Geometry check sheet. Reference: the model listing, model coordinates, mm. Face numbers are marked on the shaded views. A direction names the side the tool comes from. Coordinates: 2 decimals unless noted, no trailing zeros. Write each loop counter-clockwise with the first axis right and the second up, starting at its lowest first coordinate (ties: lowest second). Pieces come first, ordered by that corner, then holes. Notation, with made-up numbers: (30, 66.5) -> (67, 66.5) arc R6 cw to (67, 74.5) -> close; hole circle Ø5 at (35, 23). An arc over 180 degrees is marked (long way). One line per question, with ' | ' between items.
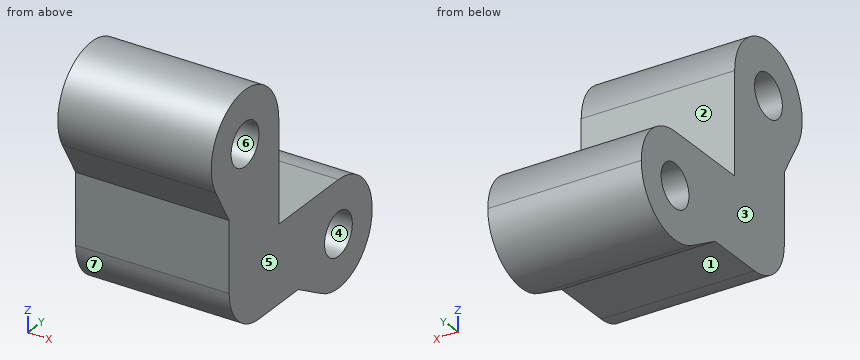
from build123d import *

# Parameters (mm, degrees)
F0_R     = 1.4
F1_DEPTH = 10
F2_R     = 3


with BuildPart() as f1:
    # F0 (on Right) → F1 (new body)
    with BuildSketch(Plane.YZ):
        with BuildLine():
            ThreePointArc((-1.7, -2.944486), (1.7, -2.944486), (3.4, 0))
            ThreePointArc((3.4, 0), (2.404163, 2.404163), (0, 3.4))
            ThreePointArc((0, 3.4), (-3.284148, 0.879985), (-1.7, -2.944486))
        make_face()
        Circle(F0_R, mode=Mode.SUBTRACT)
        with BuildLine():
            ThreePointArc((-1.7, -2.944486), (-3.284148, 0.879985), (0, 3.4))
            Line((0, 3.4), (-6, 3.4))
            Line((-6, 3.4), (-6, 10))
            ThreePointArc((-6, 10), (-8.520015, 6.715852), (-12.344486, 8.3))
            Line((-12.344486, 8.3), (-11, 5.971281))
            Line((-11, 5.971281), (-11, -1.6))
            Line((-11, -1.6), (-4.028719, -1.6))
            Line((-4.028719, -1.6), (-1.7, -2.944486))
        make_face()
        with BuildLine():
            ThreePointArc((-12.344486, 8.3), (-8.520015, 6.715852), (-6, 10))
            ThreePointArc((-6, 10), (-10.279985, 13.284148), (-12.344486, 8.3))
        make_face()
        with Locations((-9.4, 10)):
            Circle(F0_R, mode=Mode.SUBTRACT)
    extrude(amount=F1_DEPTH)

    # F2
    f2_edges = [f1.edges().sort_by_distance(p)[0] for p in [
        (5, -11, -1.6),
    ]]
    fillet(f2_edges, radius=F2_R)


solid = f1.part
1. Cross-section at B-B on y = -10.5. Record the boundary of the cut face in (x, z).
Worked answers:
outline: (0, -0.26) -> (10, -0.26) -> (10, 9.13) -> (0, 9.13) -> close; (0, 10.87) -> (10, 10.87) -> (10, 13.22) -> (0, 13.22) -> close
2. Cross-section at D-D on z = 4.5. Record the boundary of the cut face in (x, y), and give its area (3 significant figures).
Worked answers:
outline: (0, -11) -> (10, -11) -> (10, -6) -> (0, -6) -> close | area: 50.0 mm²
3. Go/stop test with flat-tipped pins: P1, Ø5, axis at x = 6, z = 2.5, coming from the -Y side; P2, Ø1.8, axis at x = 2.5, y = -3, coming from the +Z side; P3, Ø4.5, axis at x = 3, y = -7, coming from the -Z side; P4, Ø1, axis at x = 2, y = -0.5, coming from the -Z side. Record where each tip stops, or that it passes through.
Worked answers:
P1: y = -11 | P2: z = 3.4 | P3: z = -1.6 | P4: z = -3.4
4. Mould release check, pull along Y, two halves, no side actions. Record for the marked faces 4, 5, 6 and 7: released by +Y, released by -Y, zero draft, split by the parting line, or undercut.
Worked answers:
face 4: undercut | face 5: zero draft | face 6: undercut | face 7: released by -Y
5. Material ranges on line 1 (Z direction, x = 7.5, y = 0); line 2 (Y direction, x = 4.25, z = 4.5); line 3 (Z direction, x = 4, y = -9.4), recorded low to high. Write a range as from..to.
Worked answers:
line 1: -3.4..-1.4, 1.4..3.4 | line 2: -11..-6 | line 3: -1.25..8.6, 11.4..13.4
6. Tool access check on the marked faces 1, 2 and 3. Record the directions out of +Z, -Z, +X, -X, +Y, -Y that give a thin tool (end or side, any length) a straight path to the whole face; none if there is none.
Worked answers:
face 1: -Z, +X, -X, -Y | face 2: +Z, +X, -X, +Y | face 3: +Z, -Z, -X, +Y, -Y
7. Cross-section at A-A on x = 4.75. Record the boundary of the cut face in (y, z).
Worked answers:
outline: (-12.34, 8.3) -> (-11, 5.97) -> (-11, 1.4) arc R3 ccw to (-8, -1.6) -> (-4.03, -1.6) -> (-1.7, -2.94) arc R3.4 ccw (long way) to (0, 3.4) -> (-6, 3.4) -> (-6, 10) arc R3.4 ccw (long way) to start; hole circle Ø2.8 at (-9.4, 10); hole circle Ø2.8 at (0, 0)
8. Cross-section at C-C on z = 1. Record the boundary of the cut face in (x, y), and give its area (3 significant figures).
Worked answers:
outline: (0, -10.97) -> (10, -10.97) -> (10, -0.98) -> (0, -0.98) -> close; (0, 0.98) -> (10, 0.98) -> (10, 3.25) -> (0, 3.25) -> close | area: 123 mm²
